from build123d import *

# Parameters (mm, degrees)
BOSS_EXTRU_1_DEPTH      = 0.5
ESQUISSE2_W             = 1
ESQUISSE2_H             = 5
BOSS_EXTRU_2_DEPTH      = 11
ESQUISSE6_R             = 1
ENL_V_MAT_EXTRU_3_DEPTH = 11
ESQUISSE7_R             = 0.75
ENL_V_MAT_EXTRU_4_DEPTH = 11


with BuildPart() as part:
    # Esquisse1 → Boss.-Extru.1 (new body)
    with BuildSketch(Plane.XY):
        Polygon((3, 5), (24.608143501, 5), (24.608143501, 28), (3, 28), (3, 33), (0, 33), (0, 0), (3, 0), align=None)
    extrude(amount=BOSS_EXTRU_1_DEPTH)

    # Esquisse2 → Boss.-Extru.2 (add)
    with BuildSketch(Plane.XY.offset(0.5)):
        with Locations((0.5, 30.5)):
            Rectangle(ESQUISSE2_W, ESQUISSE2_H)
        with Locations((0.5, 2.5)):
            Rectangle(ESQUISSE2_W, ESQUISSE2_H)
    extrude(amount=BOSS_EXTRU_2_DEPTH)

    # Esquisse6 → Enlèv. mat.-Extru.3 (cut)
    with BuildSketch(Plane.XY.offset(0.5)):
        with Locations((22.608143501, 10)):
            Circle(ESQUISSE6_R)
        with Locations((17.608143501, 10)):
            Circle(ESQUISSE6_R)
        with Locations((12.608143501, 10)):
            Circle(ESQUISSE6_R)
        with Locations((7.608143501, 10)):
            Circle(ESQUISSE6_R)
        with Locations((2.608143501, 10)):
            Circle(ESQUISSE6_R)
        with Locations((2.608143501, 23)):
            Circle(ESQUISSE6_R)
        with Locations((7.608143501, 23)):
            Circle(ESQUISSE6_R)
        with Locations((12.608143501, 23)):
            Circle(ESQUISSE6_R)
        with Locations((17.608143501, 23)):
            Circle(ESQUISSE6_R)
        with Locations((22.608143501, 23)):
            Circle(ESQUISSE6_R)
    extrude(amount=-ENL_V_MAT_EXTRU_3_DEPTH, mode=Mode.SUBTRACT)

    # Esquisse7 → Enlèv. mat.-Extru.4 (cut)
    with BuildSketch(Plane.ZY):
        with Locations((6.5, 31)):
            Circle(ESQUISSE7_R)
        with Locations(Location((6.5, 2, 0), (0, 0, 270))):
            Circle(ESQUISSE7_R)
    extrude(amount=-ENL_V_MAT_EXTRU_4_DEPTH, mode=Mode.SUBTRACT)


solid = part.part
Geometry: final body of the model. Coordinates: model frame, mm. A direction names the side the tool comes from. Give positions to 0.01 mm unless a question says otherwise; leave off trailing zeros. Write each loop counter-clockwise with the first axis right and the second up, starting at its lowest first coordinate (ties: lowest second). Pieces come first, ordered by that corner, then holes. Notation, with made-up numbers: M 54,74.5 L 75,74.5 A22 ccw 75,105.5 Z; hole C 37,85 d6. An arc over 180 degrees is marked long. Answer in a Markdown table with one row per item. Add a question column.
(1) First-contact query: pin 1 (1.2 mm diameter, centred on x = 22.61, y = 10, fed in from -Z); pin 2 (4 mm diameter, centred on y = 31, z = 7.5, fed in from +X); pin 3 (0.6 mm diameter, centred on y = 30.5, z = 0.5, fed in from +X); pin 4 (1 mm diameter, centred on x = 22, y = 24.5, fed in from +Z). Flat tips, straight axial feed; report the tip coordinate or a pass-through.
(2) Section C-C on x = 22.25. Return loops of the section in (y, z).
(3) Section A-A on z = 9.5. Return loops of the section in (x, y), and give its area (3 significant figures).
(4) Mould query, pull axis Z, two halves, no side actions, for faces 4 (the cylindrical face through (2.48, 10.99, 0.25)), 5 (the flat face through (0.5, 2.5, 11.5)), 6 (the cylindrical face through (0.493, 1.285, 6.725)). Classes: +Z half, -Z half, draft (parallel to the pull), parting line (faces both ways), or undercut.
(5) Section D-D on y = 10. Return loops of the section in (x, z), and give its area (3 significant figures).
(6) Ray query, line 1 (Z direction, x = 12.5, y = 5.5); line 2 (Z direction, x = 0.25, y = 2); line 3 (X direction, y = 29, z = 4.5). Return the intervals inside material, ascending.
(7) Reachability of faces 1 (the flat face through (0.5, 28, 5.9)), 2 (the flat face through (1, 30, 6)), 3 (the cylindrical face through (23.56, 10.3, 0.25)) from +Z, -Z, +X, -X, +Y, -Y: full face, straight path, thin tool, end or side. Return the list, or none.
(8) Section B-B on y = 2. Return loops of the section in (x, z), and give its area (3 significant figures).
Result set:
| question | item | result |
|---|---|---|
| 1 | pin 1 | passes through |
| 1 | pin 2 | stops at x = 1 |
| 1 | pin 3 | stops at x = 3 |
| 1 | pin 4 | stops at z = 0.5 |
| 2 | outline | M 5,0 L 9.07,0 L 9.07,0.5 L 5,0.5 Z; M 10.93,0 L 22.07,0 L 22.07,0.5 L 10.93,0.5 Z; M 23.93,0 L 28,0 L 28,0.5 L 23.93,0.5 Z |
| 3 | outline | M 0,0 L 1,0 L 1,5 L 0,5 Z; M 0,28 L 1,28 L 1,33 L 0,33 Z |
| 3 | area | 10.0 mm^2 |
| 4 | face 4 | draft |
| 4 | face 5 | +Z half |
| 4 | face 6 | undercut |
| 5 | outline | M 0,0 L 1.61,0 L 1.61,0.5 L 0,0.5 Z; M 3.61,0 L 6.61,0 L 6.61,0.5 L 3.61,0.5 Z; M 8.61,0 L 11.61,0 L 11.61,0.5 L 8.61,0.5 Z; M 13.61,0 L 16.61,0 L 16.61,0.5 L 13.61,0.5 Z; M 18.61,0 L 21.61,0 L 21.61,0.5 L 18.61,0.5 Z; M 23.61,0 L 24.61,0 L 24.61,0.5 L 23.61,0.5 Z |
| 5 | area | 7.30 mm^2 |
| 6 | line 1 | z = 0 to 0.5 |
| 6 | line 2 | z = 0 to 5.75, 7.25 to 11.5 |
| 6 | line 3 | x = 0 to 1 |
| 7 | face 1 | +Z, +X, -X |
| 7 | face 2 | +Z, +X, +Y, -Y |
| 7 | face 3 | +Z, -Z |
| 8 | outline | M 0,0 L 3,0 L 3,0.5 L 1,0.5 L 1,5.75 L 0,5.75 Z; M 0,7.25 L 1,7.25 L 1,11.5 L 0,11.5 Z |
| 8 | area | 11.0 mm^2 |
